```python
from build123d import *

# Parameters (mm, degrees)
SKETCH1_W                = 151
SKETCH1_H                = 61
SKETCH1_W_2              = 143
SKETCH1_H_2              = 53
BOSS_EXTRUDE1_DEPTH      = 20.25
SKETCH2_W                = 143
SKETCH2_H                = 53
BOSS_EXTRUDE2_DEPTH      = 3
SKETCH7_W                = 53
SKETCH7_H                = 37.5
CUT_EXTRUDE3_DEPTH       = 4
SKETCH9_W                = 147
SKETCH9_H                = 53
BOSS_EXTRUDE3_DEPTH      = 3
CUT_EXTRUDE4_REACH       = 92.944
SKETCH10_R               = 1.6
SKETCH12_R               = 1.55
CUT_EXTRUDE6_DEPTH       = 100.152975245
SKETCH13_W               = 7
SKETCH13_H               = 19.36
BOSS_EXTRUDE4_DEPTH      = 2
SKETCH16_R               = 1.6
CUT_EXTRUDE7_DEPTH       = 10
SKETCH17_W               = 7
SKETCH17_H               = 15
SKETCH17_R               = 2
BOSS_EXTRUDE5_DEPTH      = 3
SKETCH18_R               = 1.6
CUT_EXTRUDE8_DEPTH       = 10
SKETCH19_W               = 25
SKETCH19_H               = 12
CUT_EXTRUDE9_DEPTH       = 105.834164756
SKETCH20_W               = 7
SKETCH20_H               = 61
BOSS_EXTRUDE6_DEPTH      = 8
CUT_EXTRUDE10_REACH      = 96.336
SKETCH21_R               = 1.6
CUT_EXTRUDE11_DEPTH      = 91.550826059
CUT_EXTRUDE11_DEPTH_BACK = 91.550826059
SKETCH22_W               = 90.903507757
SKETCH22_H               = 73.955491088


with BuildPart() as part:
    # Sketch1 → Boss-Extrude1 (new, symmetric)
    with BuildSketch(Plane(origin=(0, 0, 0), x_dir=(1, 0, 0), z_dir=(0, 1, 0))):
        Rectangle(SKETCH1_W, SKETCH1_H)
        Rectangle(SKETCH1_W_2, SKETCH1_H_2, mode=Mode.SUBTRACT)
    extrude(amount=BOSS_EXTRUDE1_DEPTH, both=True)

    # Sketch2 → Boss-Extrude2 (add)
    with BuildSketch(Plane.XZ.offset(20.25)):
        Rectangle(SKETCH2_W, SKETCH2_H)
    extrude(amount=-BOSS_EXTRUDE2_DEPTH)

    # Sketch7 → Cut-Extrude3 (cut)
    with BuildSketch(Plane(origin=(75.5, 0, 0), x_dir=(0, 0, -1), z_dir=(1, 0, 0))):
        with Locations((0, 1.5)):
            Rectangle(SKETCH7_W, SKETCH7_H)
    extrude(amount=-CUT_EXTRUDE3_DEPTH, mode=Mode.SUBTRACT)

    # Sketch9 → Boss-Extrude3 (add)
    with BuildSketch(Plane(origin=(0, 20.25, 0), x_dir=(1, 0, 0), z_dir=(0, 1, 0))):
        with Locations((2, 0)):
            Rectangle(SKETCH9_W, SKETCH9_H)
    extrude(amount=-BOSS_EXTRUDE3_DEPTH)

    # Sketch10 → Cut-Extrude4 (cut, up to next)
    with BuildSketch(Plane(origin=(0, 20.25, 0), x_dir=(1, 0, 0), z_dir=(0, 1, 0)), mode=Mode.PRIVATE) as cut_extrude4_sk1:
        with Locations(Location((60, 24.1, 0), (0, 0, 270))):
            Circle(SKETCH10_R)
    cut_extrude4_tool1 = extrude(cut_extrude4_sk1.sketch, amount=-CUT_EXTRUDE4_REACH, mode=Mode.PRIVATE) & part.part
    # Sketch10 → Cut-Extrude4 (cut, up to next)
    with BuildSketch(Plane(origin=(0, 20.25, 0), x_dir=(1, 0, 0), z_dir=(0, 1, 0)), mode=Mode.PRIVATE) as cut_extrude4_sk2:
        with Locations(Location((60, -24.1, 0), (0, 0, 90))):
            Circle(SKETCH10_R)
    cut_extrude4_tool2 = extrude(cut_extrude4_sk2.sketch, amount=-CUT_EXTRUDE4_REACH, mode=Mode.PRIVATE) & part.part
    # Sketch10 → Cut-Extrude4 (cut, up to next)
    with BuildSketch(Plane(origin=(0, 20.25, 0), x_dir=(1, 0, 0), z_dir=(0, 1, 0)), mode=Mode.PRIVATE) as cut_extrude4_sk3:
        with Locations(Location((-6.04, 21, 0), (0, 0, 270))):
            Circle(SKETCH10_R)
    cut_extrude4_tool3 = extrude(cut_extrude4_sk3.sketch, amount=-CUT_EXTRUDE4_REACH, mode=Mode.PRIVATE) & part.part
    # Sketch10 → Cut-Extrude4 (cut, up to next)
    with BuildSketch(Plane(origin=(0, 20.25, 0), x_dir=(1, 0, 0), z_dir=(0, 1, 0)), mode=Mode.PRIVATE) as cut_extrude4_sk4:
        with Locations(Location((-6.04, -21, 0), (0, 0, 90))):
            Circle(SKETCH10_R)
    cut_extrude4_tool4 = extrude(cut_extrude4_sk4.sketch, amount=-CUT_EXTRUDE4_REACH, mode=Mode.PRIVATE) & part.part
    add(cut_extrude4_tool1.solids().sort_by_distance((60, 20.25, -24.1))[0], mode=Mode.SUBTRACT)
    add(cut_extrude4_tool2.solids().sort_by_distance((60, 20.25, 24.1))[0], mode=Mode.SUBTRACT)
    add(cut_extrude4_tool3.solids().sort_by_distance((-6.04, 20.25, -21))[0], mode=Mode.SUBTRACT)
    add(cut_extrude4_tool4.solids().sort_by_distance((-6.04, 20.25, 21))[0], mode=Mode.SUBTRACT)

    # Sketch12 → Cut-Extrude6 (cut, through all)
    with BuildSketch(Plane.XY.offset(30.5)):
        with Locations((67.445205237, 4.65)):
            Circle(SKETCH12_R)
        with Locations((67.445205237, -4.65)):
            Circle(SKETCH12_R)
        with Locations((17.545205237, 4.65)):
            Circle(SKETCH12_R)
        with Locations((17.545205237, -4.65)):
            Circle(SKETCH12_R)
    extrude(amount=-CUT_EXTRUDE6_DEPTH, mode=Mode.SUBTRACT)

    # Sketch13 → Boss-Extrude4 (add)
    with BuildSketch(Plane.XY.offset(17)):
        with Locations((-69.37, 29.93)):
            Rectangle(SKETCH13_W, SKETCH13_H)
    boss_extrude4 = extrude(amount=BOSS_EXTRUDE4_DEPTH)

    # Sketch16 → Cut-Extrude7 (cut)
    with BuildSketch(Plane.XY.offset(19)):
        with Locations((-69.262241782, 24.85)):
            Circle(SKETCH16_R)
        with Locations((-69.262241782, 34.85)):
            Circle(SKETCH16_R)
    cut_extrude7 = extrude(amount=-CUT_EXTRUDE7_DEPTH, mode=Mode.SUBTRACT)

    # Mirror1: Boss-Extrude4, Cut-Extrude7 across plane
    add(boss_extrude4.mirror(Plane(origin=(-44.87, 0, 0), x_dir=(0, 0, 1), z_dir=(1, 0, 0))))
    add(cut_extrude7.mirror(Plane(origin=(-44.87, 0, 0), x_dir=(0, 0, 1), z_dir=(1, 0, 0))), mode=Mode.SUBTRACT)

    # Sketch17 → Boss-Extrude5 (add)
    with BuildSketch(Plane(origin=(0, 0, -30.5), x_dir=(-1, 0, 0), z_dir=(0, 0, -1))):
        with Locations((55.31, 27.75)):
            Rectangle(SKETCH17_W, SKETCH17_H)
        with Locations((55.31, 30.15)):
            Circle(SKETCH17_R, mode=Mode.SUBTRACT)
    extrude(amount=-BOSS_EXTRUDE5_DEPTH)

    # Sketch18 → Cut-Extrude8 (cut)
    with BuildSketch(Plane.XZ.offset(20.25)):
        with Locations(Location((-56.5, 20, 0), (0, 0, 270))):
            Circle(SKETCH18_R)
        with Locations(Location((-56.5, -20, 0), (0, 0, 270))):
            Circle(SKETCH18_R)
    extrude(amount=-CUT_EXTRUDE8_DEPTH, mode=Mode.SUBTRACT)

    # Sketch19 → Cut-Extrude9 (cut, through all)
    with BuildSketch(Plane.XY.offset(30.5)):
        with Locations((-56, -11.25)):
            Rectangle(SKETCH19_W, SKETCH19_H)
    extrude(amount=-CUT_EXTRUDE9_DEPTH, mode=Mode.SUBTRACT)

    # Sketch20 → Boss-Extrude6 (add)
    with BuildSketch(Plane(origin=(0, 20.25, 0), x_dir=(1, 0, 0), z_dir=(0, 1, 0))):
        with Locations((8, 0)):
            Rectangle(SKETCH20_W, SKETCH20_H)
    boss_extrude6 = extrude(amount=BOSS_EXTRUDE6_DEPTH)

    # Sketch21 → Cut-Extrude10 (cut, up to next)
    with BuildSketch(Plane.ZY.offset(-4.5), mode=Mode.PRIVATE) as cut_extrude10_sk1:
        with Locations((-20, 24.25)):
            Circle(SKETCH21_R)
    cut_extrude10_tool1 = extrude(cut_extrude10_sk1.sketch, amount=-CUT_EXTRUDE10_REACH, mode=Mode.PRIVATE) & part.part
    # Sketch21 → Cut-Extrude10 (cut, up to next)
    with BuildSketch(Plane.ZY.offset(-4.5), mode=Mode.PRIVATE) as cut_extrude10_sk2:
        with Locations((20, 24.25)):
            Circle(SKETCH21_R)
    cut_extrude10_tool2 = extrude(cut_extrude10_sk2.sketch, amount=-CUT_EXTRUDE10_REACH, mode=Mode.PRIVATE) & part.part
    cut_extrude10_1 = cut_extrude10_tool1.solids().sort_by_distance((4.5, 24.25, -20))[0]
    add(cut_extrude10_1, mode=Mode.SUBTRACT)
    cut_extrude10_2 = cut_extrude10_tool2.solids().sort_by_distance((4.5, 24.25, 20))[0]
    add(cut_extrude10_2, mode=Mode.SUBTRACT)
    cut_extrude10 = cut_extrude10_1 + cut_extrude10_2  # Cut-Extrude10 as one shape, for the pattern or mirror that repeats it

    # Mirror2: Boss-Extrude6, Cut-Extrude10 across plane
    add(boss_extrude6.mirror(Plane.ZX))
    add(cut_extrude10.mirror(Plane.ZX), mode=Mode.SUBTRACT)

    # Sketch22 → Cut-Extrude11 (cut, two sides: drawn at the far end of the back side and taken through both)
    with BuildSketch(Plane(origin=(0, 0, 0), x_dir=(1, 0, 0), z_dir=(0, 1, 0)).offset(-CUT_EXTRUDE11_DEPTH_BACK)):
        with Locations((-37.451753878, 4.7681e-05)):
            Rectangle(SKETCH22_W, SKETCH22_H)
    extrude(amount=CUT_EXTRUDE11_DEPTH + CUT_EXTRUDE11_DEPTH_BACK, mode=Mode.SUBTRACT)


solid = part.part
```
Could you check a few things on this model? Use its own coordinates, in mm. A direction names the side the tool comes from. Round coordinates to 2 decimals unless told otherwise and drop trailing zeros. Order: outer loops, then holes, each group sorted by start corner. A loop starts at its lowest first (then second) coordinate and runs counter-clockwise, first axis right, second up. Notation, with made-up numbers: M -3,72.5 L 44,72.5 A17 cw 44,90.5 Z; hole C 75,-26.5 d9. An arc over 180 degrees is marked long. One line per question, with ' | ' between items. Start each with the question number.
(1) Suppose I cut it at B-B on x = 60. List the corners of the cut face in (y, z) for me.
(2) Suppose I cut it at C-C on x = 42. List the corners of the cut face in (y, z) for me, then the cut area to 3 significant figures.
(3) For faces 4 (the face through (43, 20.25, 0)), 5 (the face through (42, -17.25, 0)), 6 (the face through (18.98, -5.24, -28.47)), 7 (the face through (61.35, 18.77, -23.24)), which set-ups out of +Z, -Z, +X, -X, +Y, -Y let a thin tool reach every point of the face, with its end or its side?
(4) Suppose I cut it at D-D on z = -20. List the corners of the cut face in (x, y) for me.
(5) Suppose I cut it at A-A on y = 0.5. List the corners of the cut face in (x, z) for me, then the cut area to 3 significant figures.
(6) Thinking about a two-plate mould opening in X: for faces 1 (the face through (42, 0, -26.5)), 2 (the face through (11.5, 24, 0)), 3 (the face through (18.98, 4.06, -28.47)), which applies, +X half, -X half, draft (parallel to the pull), parting line (faces both ways), or undercut?
(7) For P1, Ø8, axis at y = -13.5, z = 15.5, coming from the -X side; P2, Ø1.9, axis at x = 60, z = -24.1, coming from the +Y side; P3, Ø3, axis at x = 63.5, z = -18.5, coming from the +Y side; P4, Ø1.5, axis at x = 53, z = -8, coming from the -Y side, each with a flat end and sliding along its axis, tell me the tip position at first contact or that it passes through.
(8) Please list where these lines run through material, in increasing order: line 1 along Y through (x, z) = (9.8, -20); line 2 along Z through (x, y) = (9, -24); line 3 along Y through (x, z) = (13, -20.5).
Geometry results:
1) outline: M -20.25,-30.5 L 20.25,-30.5 L 20.25,-25.7 L 17.25,-25.7 L 17.25,-26.5 L -17.25,-26.5 L -17.25,26.5 L 17.25,26.5 L 17.25,25.7 L 20.25,25.7 L 20.25,30.5 L -20.25,30.5 Z; M 17.25,-22.5 L 20.25,-22.5 L 20.25,22.5 L 17.25,22.5 Z
2) outline: M -20.25,-30.5 L 20.25,-30.5 L 20.25,30.5 L -20.25,30.5 Z; hole M -17.25,-26.5 L 17.25,-26.5 L 17.25,26.5 L -17.25,26.5 Z | area: 642 mm²
3) face 4: +Z, -Z, +X, +Y | face 5: +X, -X | face 6: +Z, -Z | face 7: +Y
4) outline: M 8,-28.25 L 11.5,-28.25 L 11.5,-25.85 L 8,-25.85 Z; M 8,-22.65 L 11.5,-22.65 L 11.5,-20.25 L 75.5,-20.25 L 75.5,-17.25 L 8,-17.25 Z; M 8,17.25 L 75.5,17.25 L 75.5,20.25 L 11.5,20.25 L 11.5,22.65 L 8,22.65 Z; M 8,25.85 L 11.5,25.85 L 11.5,28.25 L 8,28.25 Z
5) outline: M 8,-30.5 L 75.5,-30.5 L 75.5,-26.5 L 8,-26.5 Z; M 8,26.5 L 75.5,26.5 L 75.5,30.5 L 8,30.5 Z | area: 540 mm²
6) face 1: draft | face 2: +X half | face 3: undercut
7) P1: x = 8 | P2: y = -17.25 | P3: y = 20.25 | P4: y = -20.25
8) line 1: -28.25 to -25.85, -22.65 to -17.25, 17.25 to 22.65, 25.85 to 28.25 | line 2: -30.5 to -21.58, -18.42 to 18.42, 21.58 to 30.5 | line 3: -20.25 to -17.25, 17.25 to 20.25
